Input: part model. Units: mm. Frame: model coordinates. A direction names the side the tool comes from. Round coordinates to 2 decimals unless told otherwise and drop trailing zeros. Loops run counter-clockwise (first coordinate to the right, second up) from the corner with the lowest first, then second, coordinate; pieces in that order, holes last. Notation, with made-up numbers: M -30,-33 L 15,-33 A38 cw 15,5 Z; hole C 58.5,-33.5 d7. An arc over 180 degrees is marked long. Return JSON: item names as keys, results as strings. Group by question number.
1) Section D-D (y = 21). Output: boundary loops of the cut face in (x, z).
2) Mould query, pull axis X, two halves, no side actions, for faces 6 (the face through (17.346, 47.169, -8.135)), 7 (the face through (12, 24.405, -17)), 8 (the face through (7.07, 38.743, -16.993)). Classes: +X half, -X half, draft (parallel to the pull), parting line (faces both ways), or undercut.
3) Section C-C (x = 7.5). Count the separate pieces of the cut face and the enclosed holes in it, plus the area to 3 significant figures.
4) Material intervals for line 1 (Y direction, x = 7.5, z = 0.4); line 2 (Y direction, x = 7.5, z = 1.1); line 3 (Z direction, x = 1.5, y = 48.5), sorted ascending. Write a range as from..to.
5) Section B-B (z = -8.75). Output: boundary loops of the cut face in (x, y).
6) Section A-A (y = 31.68). Output: boundary loops of the cut face in (x, z).
7) Contact query for flat-ended pins moving along their axis: P1, Ø2, axis at y = 37, z = -11, coming from the +X side; P2, Ø8, axis at y = 34, z = -5.5, coming from the -X side; P3, Ø10, axis at y = 40, z = -6, coming from the +X side; P4, Ø1.6, axis at x = 7, z = -15, coming from the -Y side. Output: stop coordinate, or through.
8) Access query for faces 1 (the face through (17.547, 19, -8)), 2 (the face through (15.126, 25.436, -8.134)), 3 (the face through (6, 39, -17.5)), 4 (the face through (17, 34, -8)), 5 (the face through (15.483, 19, -8)). Directions: +Z, -Z, +X, -X, +Y, -Y. A direction counts if a zero-diameter tool reaches every point of the face in a straight line with its end or side. Return the directions, or none.
from build123d import *

# Parameters (mm, degrees)
BOSS_EXTRUDE1_START = 2
BOSS_EXTRUDE1_DEPTH = 20.5
CUT_EXTRUDE1_DEPTH  = 8.25
SKETCH4_R           = 1.984375
CUT_EXTRUDE2_DEPTH  = 60.042444086
SKETCH5_R           = 3
CUT_EXTRUDE3_DEPTH  = 1
SKETCH6_R           = 3.444339348
CUT_EXTRUDE4_DEPTH  = 1
FILLET1_R           = 3
SKETCH9_W           = 2.063859561
SKETCH9_H           = 8.45
BOSS_EXTRUDE4_DEPTH = 9
BOSS_EXTRUDE5_DEPTH = 8.45
CUT_EXTRUDE5_DEPTH  = 59.145478277
FILLET3_R           = 3
SKETCH12_W          = 4.417525097
SKETCH12_H          = 36.817204543
CUT_EXTRUDE6_DEPTH  = 58.470832985


with BuildPart() as part:
    # Sketch1 → Boss-Extrude1 (new body)
    with BuildSketch(Plane.XY.offset(BOSS_EXTRUDE1_START)):
        with BuildLine():
            Line((17, 26.68), (17, 41.483303111))
            ThreePointArc((17, 41.483303111), (17.205901326, 42.903379834), (17.80664716, 44.206498286))
            Line((17.80664716, 44.206498286), (22.074645554, 50.778639479))
            Line((22.074645554, 50.778639479), (1.804469576, 50.778639479))
            Line((1.804469576, 50.778639479), (0.80664716, 49.2421277))
            ThreePointArc((0.80664716, 49.2421277), (0.205901326, 47.939009249), (0, 46.518932525))
            Line((0, 46.518932525), (0, 24.405491581))
            Line((0, 24.405491581), (17.547291672, 24.405491581))
            ThreePointArc((17.547291672, 24.405491581), (17.138748019, 25.51028671), (17, 26.68))
        make_face()
    extrude(amount=-BOSS_EXTRUDE1_DEPTH)

    # Sketch2 → Cut-Extrude1 (cut, symmetric)
    with BuildSketch(Plane.XY.offset(-8.25)):
        with BuildLine():
            Line((1.804469576, 50.778639479), (0.80664716, 49.2421277))
            ThreePointArc((0.80664716, 49.2421277), (0.205901326, 47.939009249), (0, 46.518932525))
            Line((0, 46.518932525), (0, 24.405491581))
            Line((0, 24.405491581), (15.483432111, 24.405491581))
            ThreePointArc((15.483432111, 24.405491581), (15.122355105, 25.45104141), (15, 26.550395893))
            Line((15, 26.550395893), (15, 42.075730101))
            ThreePointArc((15, 42.075730101), (15.205901326, 43.495806824), (15.80664716, 44.798925276))
            Line((15.80664716, 44.798925276), (19.689918969, 50.778639479))
            Line((19.689918969, 50.778639479), (1.804469576, 50.778639479))
        make_face()
    extrude(amount=CUT_EXTRUDE1_DEPTH, both=True, mode=Mode.SUBTRACT)

    # Sketch4 → Cut-Extrude2 (cut, through all)
    with BuildSketch(Plane.XY.offset(2)):
        with Locations((7.5, 40.68)):
            Circle(SKETCH4_R)
        with Locations((7.5, 31.68)):
            Circle(SKETCH4_R)
    extrude(amount=-CUT_EXTRUDE2_DEPTH, mode=Mode.SUBTRACT)

    # Sketch5 → Cut-Extrude3 (cut)
    with BuildSketch(Plane.XY.offset(2)):
        with Locations((7.5, 40.68)):
            Circle(SKETCH5_R)
        with Locations((7.5, 31.68)):
            Circle(SKETCH5_R)
    extrude(amount=-CUT_EXTRUDE3_DEPTH, mode=Mode.SUBTRACT)

    # Sketch6 → Cut-Extrude4 (cut)
    with BuildSketch(Plane(origin=(0, 0, -18.5), x_dir=(-1, 0, 0), z_dir=(0, 0, -1))):
        with Locations((-7.5, 40.68)):
            Circle(SKETCH6_R)
        with Locations((-7.5, 31.68)):
            Circle(SKETCH6_R)
    extrude(amount=-CUT_EXTRUDE4_DEPTH, mode=Mode.SUBTRACT)

    # Fillet1
    # the kernel refuses this fillet: 3 mm, written as the material it takes off along each edge
    with BuildSketch(Plane(origin=(22.074645554, 50.778639479, 15.813281645), x_dir=(-0.5446390350150283, -0.8386705679454232, 0), z_dir=(0, 0, -1))) as fillet1_piece_1:
        with BuildLine():
            CenterArc((FILLET1_R * 1.84177088603, FILLET1_R), FILLET1_R, 147, 123)
            Line((FILLET1_R * 1.00310031809, FILLET1_R * 1.54463903502), (0, 0))
            Line((0, 0), (FILLET1_R * 1.84177088603, 0))
        make_face()
    extrude(amount=48.126563291, mode=Mode.SUBTRACT)

    # Sketch9 → Boss-Extrude4 (add)
    with BuildSketch(Plane(origin=(0, 24.405491581, 0), x_dir=(-1, 0, 0), z_dir=(0, -1, 0))):
        with Locations((-16.515361891, 8.275)):
            Rectangle(SKETCH9_W, SKETCH9_H)
    extrude(amount=BOSS_EXTRUDE4_DEPTH)

    # Sketch10 → Boss-Extrude5 (add)
    with BuildSketch(Plane.XY.offset(-4.05)):
        Polygon((15.483432111, 15.405491581), (15.483432111, 13.961434936), (17.547291672, 15.405491581), align=None)
    extrude(amount=-BOSS_EXTRUDE5_DEPTH)

    # Sketch11 → Cut-Extrude5 (cut, through all)
    with BuildSketch(Plane.XY.offset(2)):
        with BuildLine():
            Line((17.264521068, 25.075244788), (17.547291672, 25.075244788))
            Line((17.547291672, 25.075244788), (17.547291672, 23.456711585))
            ThreePointArc((17.547291672, 23.456711585), (17.476067665, 24.278235922), (17.264521068, 25.075244788))
        make_face()
    extrude(amount=-CUT_EXTRUDE5_DEPTH, mode=Mode.SUBTRACT)

    # Fillet3
    fillet3_edges = [part.edges().sort_by_distance(p)[0] for p in [
        (0, 24.405491581, -17.5),
        (1.804469576, 50.778639479, -17.5),
        (1.804469576, 50.778639479, 1),
        (0, 24.405491581, 1),
    ]]
    fillet(fillet3_edges, radius=FILLET3_R)

    # Sketch12 → Cut-Extrude6 (cut, through all)
    with BuildSketch(Plane.ZY):
        with Locations((-19.908762549, 32.370037208)):
            Rectangle(SKETCH12_W, SKETCH12_H)
        with Locations((3.408762549, 32.370037208)):
            Rectangle(SKETCH12_W, SKETCH12_H)
    extrude(amount=-CUT_EXTRUDE6_DEPTH, mode=Mode.SUBTRACT)


solid = part.part
Returned:
{
 "1": {"outline": "M 15.48,-12.5 L 17.55,-12.5 L 17.55,-4.05 L 15.48,-4.05 Z"},
 "2": {"face 6": "-X half", "face 7": "draft", "face 8": "undercut"},
 "3": {"separate pieces": "6", "enclosed holes": "0", "area": "42.3 mm^2"},
 "4": {"line 1": "y = 24.41..29.7, 33.66..38.7, 42.66..50.78", "line 2": "y = 24.41..28.68, 34.68..37.68, 43.68..50.78", "line 3": "z = -17.7..-16.5, 0..1.2"},
 "5": {"outline": "M 15,26.55 A5 ccw 15.48,24.41 L 15.48,13.96 L 17.55,15.41 L 17.55,23.46 A4.77 ccw 17.3,24.99 A5 cw 17,26.68 L 17,41.48 A5 cw 17.81,44.21 L 19.07,46.14 A3 ccw 18.93,49.61 L 15.81,44.8 A5 ccw 15,42.08 Z"},
 "6": {"outline": "M 0,-17.7 L 4.06,-17.7 L 4.06,-17.5 L 5.52,-17.5 L 5.52,-16.5 L 0,-16.5 Z; M 0,0 L 5.52,0 L 5.52,1 L 4.5,1 L 4.5,1.2 L 0,1.2 Z; M 9.48,-17.5 L 10.94,-17.5 L 10.94,-17.7 L 17,-17.7 L 17,1.2 L 10.5,1.2 L 10.5,1 L 9.48,1 L 9.48,0 L 15,0 L 15,-16.5 L 9.48,-16.5 Z"},
 "7": {"P1": "stops at x = 17", "P2": "stops at x = 15", "P3": "stops at x = 18.32", "P4": "passes through"},
 "8": {"face 1": "+Z, -Z, +X, -Y", "face 2": "-X, -Y", "face 3": "-Z", "face 4": "+Z, -Z, +X", "face 5": "+Z, -Z, -X, -Y"}
}
